For this review, take the finished solid that the model builds, in its own axes (mm). A direction names the side the tool comes from. Coordinates: 2 decimals unless noted, no trailing zeros. Loops run counter-clockwise (first coordinate to the right, second up) from the corner with the lowest first, then second, coordinate; pieces in that order, holes last. Notation, with made-up numbers: (-17, 9) -> (19, 9) arc R27 cw to (19, 35) -> close; hole circle Ø5 at (61.5, -25.5). An arc over 180 degrees is marked (long way). Use a Markdown table: item, result.
from build123d import *

# Parameters (mm, degrees)
CROQUIS1_W              = 6
CROQUIS1_H              = 6
SALIENTE_EXTRUIR1_DEPTH = 3.5
CROQUIS2_R              = 4.5
SALIENTE_EXTRUIR2_DEPTH = 4
CROQUIS3_R              = 4
SALIENTE_EXTRUIR3_DEPTH = 6
CROQUIS4_W              = 5
CROQUIS4_H              = 5
CORTAR_EXTRUIR1_DEPTH   = 5


with BuildPart() as part:
    # Croquis1 → Saliente-Extruir1 (new body)
    with BuildSketch(Plane.XY):
        Rectangle(CROQUIS1_W, CROQUIS1_H)
    extrude(amount=SALIENTE_EXTRUIR1_DEPTH)

    # Croquis2 → Saliente-Extruir2 (add)
    with BuildSketch(Plane.XY.offset(3.5)):
        Circle(CROQUIS2_R)
    extrude(amount=SALIENTE_EXTRUIR2_DEPTH)

    # Croquis3 → Saliente-Extruir3 (add)
    with BuildSketch(Plane.XY.offset(7.5)):
        Circle(CROQUIS3_R)
    extrude(amount=SALIENTE_EXTRUIR3_DEPTH)

    # Croquis4 → Cortar-Extruir1 (cut)
    with BuildSketch(Plane.XY.offset(13.5)):
        Rectangle(CROQUIS4_W, CROQUIS4_H)
    extrude(amount=-CORTAR_EXTRUIR1_DEPTH, mode=Mode.SUBTRACT)


solid = part.part
(1) Take a section at A-A on x = 0. Write out the cut boundary in (y, z), plus the area to 3 significant figures.
Found:
| item | result |
|---|---|
| outline | (-4.5, 3.5) -> (-3, 3.5) -> (-3, 0) -> (3, 0) -> (3, 3.5) -> (4.5, 3.5) -> (4.5, 7.5) -> (4, 7.5) -> (4, 13.5) -> (2.5, 13.5) -> (2.5, 8.5) -> (-2.5, 8.5) -> (-2.5, 13.5) -> (-4, 13.5) -> (-4, 7.5) -> (-4.5, 7.5) -> close |
| area | 80.0 mm^2 |
(2) For faces 4 (the face through (0, -3, 2)), 5 (the face through (3, 0, 2)), 6 (the face through (0, 3, 2)), 7 (the face through (-0.867, -3.905, 10.458)), list the 3-axis set-ups (+Z, -Z, +X, -X, +Y, -Y) from which the entire face can be reached by the end or side of a thin tool; tool diameter is ignored.
Found:
| item | result |
|---|---|
| face 4 | -Z, +X, -X, -Y |
| face 5 | -Z, +X, +Y, -Y |
| face 6 | -Z, +X, -X, +Y |
| face 7 | +Z |
(3) For pin 1 Ø4 at (y, z) = (-2.5, 8) entering from +X; pin 2 Ø3 at (y, z) = (2.5, 3.5) entering from +X; pin 3 Ø4 at (y, z) = (1.5, 5.5) entering from -X; pin 4 Ø1.5 at (x, z) = (0.5, 11) entering from +Y, all flat-tipped, find the tip position at first contact; note any pin that passes through.
Found:
| item | result |
|---|---|
| pin 1 | stops at x = 4.46 |
| pin 2 | stops at x = 4.39 |
| pin 3 | stops at x = -4.5 |
| pin 4 | stops at y = 4 |
(4) For line 1 along Z through (x, y) = (-0.5, -0.75); line 2 along Z through (x, y) = (4, -1); line 3 along Y through (x, z) = (2, 1), list the stretches that pass through material, from the lowest coordinate up.
Found:
| item | result |
|---|---|
| line 1 | z = 0 to 8.5 |
| line 2 | z = 3.5 to 7.5 |
| line 3 | y = -3 to 3 |
(5) Take a section at C-C on z = 9.75. Write out the cut boundary in (x, y).
Found:
| item | result |
|---|---|
| outline | circle Ø8 at (0, 0); hole (-2.5, -2.5) -> (2.5, -2.5) -> (2.5, 2.5) -> (-2.5, 2.5) -> close |
(6) Take a section at D-D on z = 3. Write out the cut boundary in (x, y), plus the area to 3 significant figures.
Found:
| item | result |
|---|---|
| outline | (-3, -3) -> (3, -3) -> (3, 3) -> (-3, 3) -> close |
| area | 36.0 mm^2 |
(7) Mouldability with a two-part tool opening along X and no side actions: class faces 1 (the face through (3, 0, 13.5)), 2 (the face through (-2.5, 0, 11)), 3 (the face through (-3, 0, 2)) as pulls with the +X half, pulls with the -X half, needs draft (parallel to the pull), parting line crosses it, or undercut.
Found:
| item | result |
|---|---|
| face 1 | needs draft |
| face 2 | undercut |
| face 3 | pulls with the -X half |
